Check sheet for the modelled part. Datum: model origin and axes. Units: mm. Face numbers are marked on the shaded views. Give positions to 0.01 mm unless a question says otherwise; leave off trailing zeros. Order: outer loops, then holes, each group sorted by start corner. A loop starts at its lowest first (then second) coordinate and runs counter-clockwise, first axis right, second up.
```python
from build123d import *

# Parameters (mm, degrees)
F0_W     = 146.75
F0_H     = 155.1
F0_R     = 1.6
F1_DEPTH = 2.37
F2_W     = 1.3
F2_H     = 126
F3_DEPTH = 0.85
F4_W     = 2.5
F4_H     = 126
F5_DEPTH = 0.1
F6_W     = 8
F6_H     = 7.1
F7_DEPTH = 0.85


with BuildPart() as f1:
    # F0 (on Top) → F1 (new body)
    with BuildSketch(Plane.XY):
        Rectangle(F0_W, F0_H)
        with Locations((-67.005, -69.5325)):
            Circle(F0_R, mode=Mode.SUBTRACT)
        with Locations((67.005, -69.5325)):
            Circle(F0_R, mode=Mode.SUBTRACT)
        with Locations((-67.005, 69.5325)):
            Circle(F0_R, mode=Mode.SUBTRACT)
        with Locations((67.005, 69.5325)):
            Circle(F0_R, mode=Mode.SUBTRACT)
    extrude(amount=F1_DEPTH)

    # F2 (on face) → F3 (join)
    with BuildSketch(Plane.XY.offset(2.37)):
        with Locations((64.675, 0)):
            Rectangle(F2_W, F2_H)
        with Locations((38.275, 0)):
            Rectangle(F2_W, F2_H)
        with Locations((12.775, 0)):
            Rectangle(F2_W, F2_H)
        with Locations((-38.025, 0)):
            Rectangle(F2_W, F2_H)
        with Locations((-12.625, 0)):
            Rectangle(F2_W, F2_H)
        with Locations((-64.425, 0)):
            Rectangle(F2_W, F2_H)
    extrude(amount=F3_DEPTH)

    # F4 (on face) → F5 (join)
    with BuildSketch(Plane.XY.offset(2.37)):
        with Locations((-62.525, 0)):
            Rectangle(F4_W, F4_H)
        with Locations((-39.925, 0)):
            Rectangle(F4_W, F4_H)
        with Locations((-36.125, 0)):
            Rectangle(F4_W, F4_H)
        with Locations((-14.525, 0)):
            Rectangle(F4_W, F4_H)
        with Locations((-10.725, 0)):
            Rectangle(F4_W, F4_H)
        with Locations((10.875, 0)):
            Rectangle(F4_W, F4_H)
        with Locations((14.675, 0)):
            Rectangle(F4_W, F4_H)
        with Locations((36.375, 0)):
            Rectangle(F4_W, F4_H)
        with Locations((40.175, 0)):
            Rectangle(F4_W, F4_H)
        with Locations((62.775, 0)):
            Rectangle(F4_W, F4_H)
    extrude(amount=F5_DEPTH)

    # F6 (on face) → F7 (cut)
    with BuildSketch(Plane.XY.offset(3.22)):
        with Locations((-62.375, -54.45)):
            Rectangle(F6_W, F6_H)
        with Locations((-62.375, -42.35)):
            Rectangle(F6_W, F6_H)
        with Locations((-62.375, -30.25)):
            Rectangle(F6_W, F6_H)
        with Locations((-62.375, -18.15)):
            Rectangle(F6_W, F6_H)
        with Locations((-62.375, -6.05)):
            Rectangle(F6_W, F6_H)
        with Locations((-62.375, 6.05)):
            Rectangle(F6_W, F6_H)
        with Locations((-62.375, 18.15)):
            Rectangle(F6_W, F6_H)
        with Locations((-62.375, 30.25)):
            Rectangle(F6_W, F6_H)
        with Locations((-62.375, 42.35)):
            Rectangle(F6_W, F6_H)
        with Locations((-62.375, 54.45)):
            Rectangle(F6_W, F6_H)
        with Locations((63.375, -54.45)):
            Rectangle(F6_W, F6_H)
        with Locations((63.375, -42.35)):
            Rectangle(F6_W, F6_H)
        with Locations((63.375, -30.25)):
            Rectangle(F6_W, F6_H)
        with Locations((63.375, -18.15)):
            Rectangle(F6_W, F6_H)
        with Locations((63.375, -6.05)):
            Rectangle(F6_W, F6_H)
        with Locations((63.375, 6.05)):
            Rectangle(F6_W, F6_H)
        with Locations((63.375, 18.15)):
            Rectangle(F6_W, F6_H)
        with Locations((63.375, 30.25)):
            Rectangle(F6_W, F6_H)
        with Locations((63.375, 42.35)):
            Rectangle(F6_W, F6_H)
        with Locations((63.375, 54.45)):
            Rectangle(F6_W, F6_H)
    extrude(amount=-F7_DEPTH, mode=Mode.SUBTRACT)


solid = f1.part
```
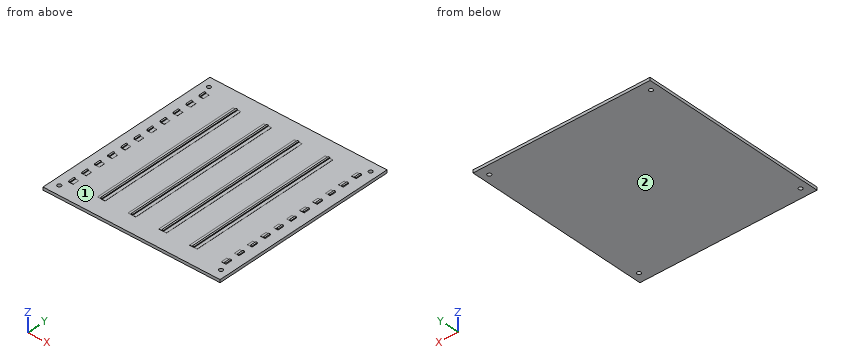
(1) Thickness scan on L1, parallel to X at y = 49.5, z = 2.7 (3 decimals); L2, parallel to X at y = -21.5, z = 2.75 (3 decimals); L3, parallel to X at y = 28, z = 2.4 (3 decimals). Record the ranges inside material, lowest first.
(2) Release check for a two-part mould opening along X. For the marked faces 1 and 2 record: released by +X, released by -X, zero draft, split by the parting line, or undercut.
(3) Go/stop test with flat-tipped pins: P1, Ø1.2, axis at x = -62.5, y = -11.5, coming from the +Z side; P2, Ø0.9, axis at y = 36.5, z = 3, coming from the +X side (3 decimals); P3, Ø1, axis at y = -41.5, z = 3, coming from the -X side (3 decimals). Record where each tip stops, or that it passes through.
(4) Sectioned sample at A-A (x = -26). Enter the section's corners in (y, z), plus the area to 3 significant figures.
Values follow:
1. L1: x = -65.075 to -63.775, -38.675 to -37.375, -13.275 to -11.975, 12.125 to 13.425, 37.625 to 38.925, 64.025 to 65.325
1. L2: x = -38.675 to -37.375, -13.275 to -11.975, 12.125 to 13.425, 37.625 to 38.925
1. L3: x = -41.175 to -34.875, -15.775 to -9.475, 9.625 to 15.925, 35.125 to 41.425
2. face 1: undercut
2. face 2: zero draft
3. P1: stops at z = 2.47
3. P2: stops at x = 65.325
3. P3: stops at x = -38.675
4. outline: (-77.55, 0) - (77.55, 0) - (77.55, 2.37) - (-77.55, 2.37) - close
4. area: 368 mm2
